Build history of the part. All positions in model axes, mm. Coordinates: 2 decimals unless noted, no trailing zeros. Loops run counter-clockwise (first coordinate to the right, second up) from the corner with the lowest first, then second, coordinate; pieces in that order, holes last.
Item 1: Cut at D-D (x = -50). List the corners of the cut face in (y, z), and give its area (3 significant figures).
Item 2: Cut at B-B (z = 0.55). List the corners of the cut face in (x, y).
Item 3: Drill centre lines: line 1 along X through (y, z) = (-42, 0.55); line 2 along X through (y, z) = (-24, 0.35) (3 decimals); line 3 along Y through (x, z) = (14, 0.8). Where is each one in solid material? Low to high.
Item 4: Cut at C-C (y = -11). List the corners of the cut face in (x, z).
Item 5: Mould opens along X. For faces 1 (the face through (51.8, 7.4, 0.5)), 2 (the face through (6.864, -17.422, 0.493)), 3 (the face through (-52.421, 3.363, 0.493)) say: released by +X, released by -X, zero draft, split by the parting line, or undercut.
Item 6: Cut at A-A (x = 10). List the corners of the cut face in (y, z).
from build123d import *

# Parameters (mm, degrees)
F0_R     = 1.25
F0_R_2   = 5.5
F0_R_3   = 5
F1_DEPTH = 1


with BuildPart() as f1:
    # F0 (on Top) → F1 (new body)
    with BuildSketch(Plane.XY):
        with BuildLine():
            Line((48.267568, 8.860779), (-44.371753, 8.860779))
            ThreePointArc((-44.371753, 8.860779), (-46.412994, 8.425134), (-48.098533, 7.194113))
            ThreePointArc((-48.098533, 7.194113), (-52.488118, 3.315719), (-57.659668, 0.56518))
            Line((-57.659668, 0.56518), (-57.659668, -3.380423))
            ThreePointArc((-57.659668, -3.380423), (-54.215032, -21.137683), (-57.658519, -38.895166))
            Line((-57.658519, -38.895166), (-57.658519, -42.844069))
            ThreePointArc((-57.658519, -42.844069), (-52.487611, -45.594512), (-48.098533, -49.472554))
            ThreePointArc((-48.098533, -49.472554), (-46.412994, -50.703575), (-44.371753, -51.139221))
            Line((-44.371753, -51.139221), (48.267568, -51.139221))
            ThreePointArc((48.267568, -51.139221), (51.803101, -49.674755), (53.267568, -46.139221))
            Line((53.267568, -46.139221), (53.267568, -22.439221))
            Line((53.267568, -22.439221), (46.782555, -22.439221))
            ThreePointArc((46.782555, -22.439221), (45.636911, -22.799861), (44.904433, -23.751721))
            ThreePointArc((44.904433, -23.751721), (37.767568, -28.739221), (30.630702, -23.751721))
            ThreePointArc((30.630702, -23.751721), (29.898224, -22.799861), (28.75258, -22.439221))
            Line((28.75258, -22.439221), (22.267568, -22.439221))
            Line((22.267568, -22.439221), (22.267568, -36.139221))
            Line((22.267568, -36.139221), (11.842568, -36.139221))
            Line((11.842568, -36.139221), (11.842568, -38.439221))
            ThreePointArc((11.842568, -38.439221), (7.156568, -42.753221), (2.842568, -38.067221))
            Line((2.842568, -38.067221), (2.842568, -36.139221))
            Line((2.842568, -36.139221), (-22.307432, -36.139221))
            Line((-22.307432, -36.139221), (-22.307432, -38.067221))
            ThreePointArc((-22.307432, -38.067221), (-26.621432, -42.753221), (-31.307432, -38.439221))
            Line((-31.307432, -38.439221), (-31.307432, -36.139221))
            Line((-31.307432, -36.139221), (-41.732432, -36.139221))
            Line((-41.732432, -36.139221), (-41.732432, -6.139221))
            Line((-41.732432, -6.139221), (-31.307432, -6.139221))
            Line((-31.307432, -6.139221), (-31.307432, -3.839221))
            ThreePointArc((-31.307432, -3.839221), (-26.621432, 0.474779), (-22.307432, -4.211221))
            Line((-22.307432, -4.211221), (-22.307432, -6.139221))
            Line((-22.307432, -6.139221), (2.842568, -6.139221))
            Line((2.842568, -6.139221), (2.842568, -4.211221))
            ThreePointArc((2.842568, -4.211221), (7.156568, 0.474779), (11.842568, -3.839221))
            Line((11.842568, -3.839221), (11.842568, -6.139221))
            Line((11.842568, -6.139221), (22.267568, -6.139221))
            Line((22.267568, -6.139221), (22.267568, -19.839221))
            Line((22.267568, -19.839221), (28.75258, -19.839221))
            ThreePointArc((28.75258, -19.839221), (29.898224, -19.47858), (30.630702, -18.526721))
            ThreePointArc((30.630702, -18.526721), (37.767568, -13.539221), (44.904433, -18.526721))
            ThreePointArc((44.904433, -18.526721), (45.636911, -19.47858), (46.782555, -19.839221))
            Line((46.782555, -19.839221), (53.267568, -19.839221))
            Line((53.267568, -19.839221), (53.267568, 3.860779))
            ThreePointArc((53.267568, 3.860779), (51.803101, 7.396313), (48.267568, 8.860779))
        make_face()
        with Locations((-38.380432, -42.839221)):
            Circle(F0_R, mode=Mode.SUBTRACT)
        with Locations((37.767568, -42.839221)):
            Circle(F0_R, mode=Mode.SUBTRACT)
        with Locations((-38.380432, 0.560779)):
            Circle(F0_R, mode=Mode.SUBTRACT)
        with Locations((37.767568, 0.560779)):
            Circle(F0_R, mode=Mode.SUBTRACT)
        with BuildLine():
            Line((22.267568, -21.139221), (22.267568, -19.839221))
            Line((22.267568, -19.839221), (22.267568, -6.139221))
            Line((22.267568, -6.139221), (11.842568, -6.139221))
            Line((11.842568, -6.139221), (11.842568, -3.839221))
            ThreePointArc((11.842568, -3.839221), (7.156568, 0.474779), (2.842568, -4.211221))
            Line((2.842568, -4.211221), (2.842568, -6.139221))
            Line((2.842568, -6.139221), (-22.307432, -6.139221))
            Line((-22.307432, -6.139221), (-22.307432, -4.211221))
            ThreePointArc((-22.307432, -4.211221), (-26.621432, 0.474779), (-31.307432, -3.839221))
            Line((-31.307432, -3.839221), (-31.307432, -6.139221))
            Line((-31.307432, -6.139221), (-41.732432, -6.139221))
            Line((-41.732432, -6.139221), (-41.732432, -36.139221))
            Line((-41.732432, -36.139221), (-31.307432, -36.139221))
            Line((-31.307432, -36.139221), (-31.307432, -38.439221))
            ThreePointArc((-31.307432, -38.439221), (-26.621432, -42.753221), (-22.307432, -38.067221))
            Line((-22.307432, -38.067221), (-22.307432, -36.139221))
            Line((-22.307432, -36.139221), (2.842568, -36.139221))
            Line((2.842568, -36.139221), (2.842568, -38.067221))
            ThreePointArc((2.842568, -38.067221), (7.156568, -42.753221), (11.842568, -38.439221))
            Line((11.842568, -38.439221), (11.842568, -36.139221))
            Line((11.842568, -36.139221), (22.267568, -36.139221))
            Line((22.267568, -36.139221), (22.267568, -22.439221))
            Line((22.267568, -22.439221), (22.267568, -21.139221))
        make_face()
        with Locations((10.917568, -21.139221)):
            Circle(F0_R_2, mode=Mode.SUBTRACT)
        with BuildLine():
            Line((53.267568, -22.439221), (53.267568, -19.839221))
            Line((53.267568, -19.839221), (46.782555, -19.839221))
            ThreePointArc((46.782555, -19.839221), (45.636911, -19.47858), (44.904433, -18.526721))
            ThreePointArc((44.904433, -18.526721), (37.767568, -13.539221), (30.630702, -18.526721))
            ThreePointArc((30.630702, -18.526721), (29.898224, -19.47858), (28.75258, -19.839221))
            Line((28.75258, -19.839221), (22.267568, -19.839221))
            Line((22.267568, -19.839221), (22.267568, -21.139221))
            Line((22.267568, -21.139221), (22.267568, -22.439221))
            Line((22.267568, -22.439221), (28.75258, -22.439221))
            ThreePointArc((28.75258, -22.439221), (29.898224, -22.799861), (30.630702, -23.751721))
            ThreePointArc((30.630702, -23.751721), (37.767568, -28.739221), (44.904433, -23.751721))
            ThreePointArc((44.904433, -23.751721), (45.636911, -22.799861), (46.782555, -22.439221))
            Line((46.782555, -22.439221), (53.267568, -22.439221))
        make_face()
        with Locations((37.767568, -21.139221)):
            Circle(F0_R_3, mode=Mode.SUBTRACT)
        with Locations((37.767568, -21.139221)):
            Circle(F0_R_3)
        with Locations((37.767568, 0.560779)):
            Circle(F0_R)
        with Locations((37.767568, -42.839221)):
            Circle(F0_R)
        with Locations((-38.380432, -42.839221)):
            Circle(F0_R)
        with Locations((-38.380432, 0.560779)):
            Circle(F0_R)
    extrude(amount=F1_DEPTH)


solid = f1.part
Filled sheet:
1. outline: (-47.56, 0) - (5.29, 0) - (5.29, 1) - (-47.56, 1) - close
1. area: 52.9 mm2
2. outline: (-57.66, -42.84) arc R25 cw to (-48.1, -49.47) arc R5 ccw to (-44.37, -51.14) - (48.27, -51.14) arc R5 ccw to (53.27, -46.14) - (53.27, 3.86) arc R5 ccw to (48.27, 8.86) - (-44.37, 8.86) arc R5 ccw to (-48.1, 7.19) arc R25 cw to (-57.66, 0.57) - (-57.66, -3.38) arc R47.5 cw to (-57.66, -38.9) - close; hole circle Ø11 at (10.92, -21.14)
3. line 1: x = -57.66 to 53.27
3. line 2: x = -54.301 to 6.22, 15.615 to 53.268
3. line 3: y = -51.14 to -25.69, -16.58 to 8.86
4. outline: (-55.31, 0) - (53.27, 0) - (53.27, 1) - (-55.31, 1) - close
5. face 1: released by +X
5. face 2: undercut
5. face 3: released by -X
6. outline: (-51.14, 0) - (-26.56, 0) - (-26.56, 1) - (-51.14, 1) - close; (-15.72, 0) - (8.86, 0) - (8.86, 1) - (-15.72, 1) - close
